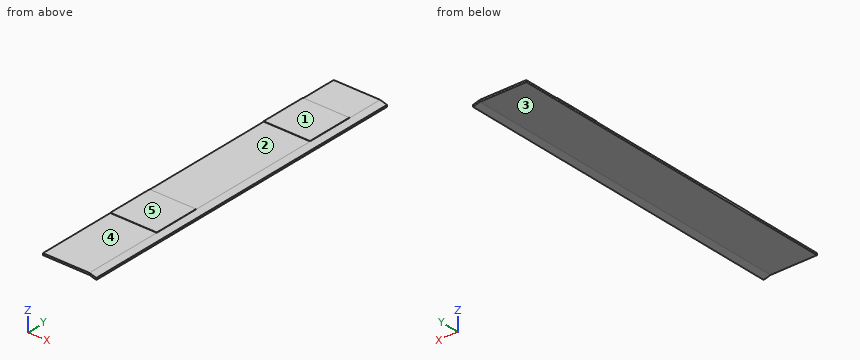
from build123d import *

# Parameters (mm, degrees)
F1_DEPTH = 1110
F2_W     = 150
F2_H     = 150
F3_DEPTH = 1


with BuildPart() as f1:
    # F0 (on Front) → F1 (new body)
    with BuildSketch(Plane.XZ):
        Polygon((150, 0), (0, 0), (0, -6), (150, -6), (172.216294, -11.952838), (172.216294, -5.952838), align=None)
    extrude(amount=F1_DEPTH)

    # F2 (on face) → F3 (join)
    with BuildSketch(Plane.XY):
        with Locations((74.428144, -192.023769)):
            Rectangle(F2_W, F2_H)
        with Locations((75, -777.969706)):
            Rectangle(F2_W, F2_H)
    extrude(amount=F3_DEPTH)


solid = f1.part
Part model, mm, in its own coordinate system. Face numbers are marked on the shaded views. A direction names the side the tool comes from. Give positions to 0.01 mm unless a question says otherwise; leave off trailing zeros. Loops run counter-clockwise (first coordinate to the right, second up) from the corner with the lowest first, then second, coordinate; pieces in that order, holes last. Notation, with made-up numbers: M 8,53.5 L 61,53.5 A20 ccw 61,79.5 Z; hole C -32.75,-6 d7. An arc over 180 degrees is marked long. Put each result on its own line as item: value. Start each with the question number.
1) Saw through at B-B (y = -240.5). List the corners of the cut face in (x, z).
2) 3-axis set-ups, long thin cutter, end or side, ignore diameter. For the marked faces 3, 4 and 5: which of +Z, -Z, +X, -X, +Y, -Y reach the whole face in a straight line?
3) Saw through at A-A (x = 86). List the corners of the cut face in (y, z), then the cut area to 3 significant figures.
4) Saw through at C-C (z = -3.75). List the corners of the cut face in (x, y).
5) Flat gauge pins, fed straight in: pin 1 (0.5 mm diameter, centred on y = -205.5, z = 0.5, fed in from +X); pin 2 (0.5 mm diameter, centred on y = -757.5, z = 0.5, fed in from +X); pin 3 (0.8 mm diameter, centred on x = 73, z = 0.5, fed in from -Y). Where does each tip first touch, or does it go through?
6) Probe probe 1 along Y at (x, z) = (70.5, 0.75); probe 2 along Z at (x, y) = (81.5, -174); probe 3 along Z at (x, y) = (146, -488.5). List the from-to ranges inside material, lowest first.
7) Pull direction Y, two halves, no side cores. Call the marked faces 1 and 2: +Y half, -Y half, draft (parallel to the pull), parting line (faces both ways), or undercut.
Numbers:
1. outline: M -0.57,0 L 0,0 L 0,-6 L 150,-6 L 172.22,-11.95 L 172.22,-5.95 L 150,0 L 149.43,0 L 149.43,1 L -0.57,1 Z
2. face 3: -Z, -X, +Y, -Y
2. face 4: +Z, +X, -X, -Y
2. face 5: +Z, +X, -X, +Y, -Y
3. outline: M -1110,-6 L 0,-6 L 0,0 L -117.02,0 L -117.02,1 L -267.02,1 L -267.02,0 L -702.97,0 L -702.97,1 L -852.97,1 L -852.97,0 L -1110,0 Z
3. area: 6,960 mm^2
4. outline: M 0,-1110 L 164,-1110 L 164,0 L 0,0 Z
5. pin 1: x = 149.43
5. pin 2: x = 150
5. pin 3: y = -852.97
6. probe 1: -852.97 to -702.97, -267.02 to -117.02
6. probe 2: -6 to 1
6. probe 3: -6 to 0
7. face 1: draft
7. face 2: undercut
